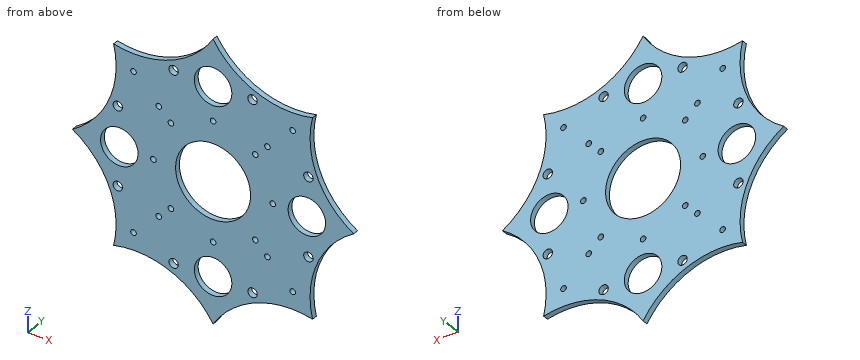
from build123d import *

# Parameters (mm, degrees)
SKETCH_1_R      = 1.5
SKETCH_1_R_2    = 20
SKETCH_1_R_3    = 2.5
SKETCH_1_R_4    = 10
EXTRUDE_2_DEPTH = 3


with BuildPart() as part:
    # 草圖1 → 填料-伸長2 (new body)
    with BuildSketch(Plane(origin=(0, 0, 0), x_dir=(1, 0, 0), z_dir=(0, 1, 0))):
        with BuildLine():
            ThreePointArc((-53.033008589, 53.033008589), (-22.961005942, 55.432771951), (0, 75))
            ThreePointArc((0, 75), (22.961005942, 55.432771951), (53.033008589, 53.033008589))
            ThreePointArc((53.033008589, 53.033008589), (55.432771951, 22.961005942), (75, 0))
            ThreePointArc((75, 0), (55.432771951, -22.961005942), (53.033008589, -53.033008589))
            ThreePointArc((53.033008589, -53.033008589), (22.961005942, -55.432771951), (0, -75))
            ThreePointArc((0, -75), (-22.961005942, -55.432771951), (-53.033008589, -53.033008589))
            ThreePointArc((-53.033008589, -53.033008589), (-55.432771951, -22.961005942), (-75, 0))
            ThreePointArc((-75, 0), (-55.432771951, 22.961005942), (-53.033008589, 53.033008589))
        make_face()
        with Locations(Location((-42.426406871, 42.426406871, 0), (0, 0, 270))):
            Circle(SKETCH_1_R, mode=Mode.SUBTRACT)
        with Locations(Location((-28.991378029, 28.991378029, 0), (0, 0, 270))):
            Circle(SKETCH_1_R, mode=Mode.SUBTRACT)
        with Locations(Location((28.991378029, -28.991378029, 0), (0, 0, 270))):
            Circle(SKETCH_1_R, mode=Mode.SUBTRACT)
        with Locations(Location((42.426406871, -42.426406871, 0), (0, 0, 270))):
            Circle(SKETCH_1_R, mode=Mode.SUBTRACT)
        with Locations(Location((42.426406871, 42.426406871, 0), (0, 0, 270))):
            Circle(SKETCH_1_R, mode=Mode.SUBTRACT)
        with Locations(Location((28.991378029, 28.991378029, 0), (0, 0, 270))):
            Circle(SKETCH_1_R, mode=Mode.SUBTRACT)
        with Locations(Location((-28.991378029, -28.991378029, 0), (0, 0, 270))):
            Circle(SKETCH_1_R, mode=Mode.SUBTRACT)
        with Locations(Location((-42.426406871, -42.426406871, 0), (0, 0, 270))):
            Circle(SKETCH_1_R, mode=Mode.SUBTRACT)
        with Locations(Location((0, 0, 0), (0, 0, 270))):
            Circle(SKETCH_1_R_2, mode=Mode.SUBTRACT)
        with Locations(Location((0, 31.819805153, 0), (0, 0, 270))):
            Circle(SKETCH_1_R, mode=Mode.SUBTRACT)
        with Locations(Location((31.819805153, 0, 0), (0, 0, 270))):
            Circle(SKETCH_1_R, mode=Mode.SUBTRACT)
        with Locations(Location((22.5, 22.5, 0), (0, 0, 270))):
            Circle(SKETCH_1_R, mode=Mode.SUBTRACT)
        with Locations(Location((0, -31.819805153, 0), (0, 0, 270))):
            Circle(SKETCH_1_R, mode=Mode.SUBTRACT)
        with Locations(Location((-22.5, -22.5, 0), (0, 0, 270))):
            Circle(SKETCH_1_R, mode=Mode.SUBTRACT)
        with Locations(Location((-31.819805153, 0, 0), (0, 0, 270))):
            Circle(SKETCH_1_R, mode=Mode.SUBTRACT)
        with Locations(Location((-22.5, 22.5, 0), (0, 0, 270))):
            Circle(SKETCH_1_R, mode=Mode.SUBTRACT)
        with Locations(Location((22.5, -22.5, 0), (0, 0, 270))):
            Circle(SKETCH_1_R, mode=Mode.SUBTRACT)
        with Locations(Location((-21.04758878, 50.813374288, 0), (0, 0, 270))):
            Circle(SKETCH_1_R_3, mode=Mode.SUBTRACT)
        with Locations(Location((21.04758878, 50.813374288, 0), (0, 0, 270))):
            Circle(SKETCH_1_R_3, mode=Mode.SUBTRACT)
        with Locations(Location((50.813374288, 21.04758878, 0), (0, 0, 270))):
            Circle(SKETCH_1_R_3, mode=Mode.SUBTRACT)
        with Locations(Location((50.813374288, -21.04758878, 0), (0, 0, 270))):
            Circle(SKETCH_1_R_3, mode=Mode.SUBTRACT)
        with Locations(Location((21.04758878, -50.813374288, 0), (0, 0, 270))):
            Circle(SKETCH_1_R_3, mode=Mode.SUBTRACT)
        with Locations(Location((-21.04758878, -50.813374288, 0), (0, 0, 270))):
            Circle(SKETCH_1_R_3, mode=Mode.SUBTRACT)
        with Locations(Location((-50.813374288, -21.04758878, 0), (0, 0, 270))):
            Circle(SKETCH_1_R_3, mode=Mode.SUBTRACT)
        with Locations(Location((-50.813374288, 21.04758878, 0), (0, 0, 270))):
            Circle(SKETCH_1_R_3, mode=Mode.SUBTRACT)
        with Locations(Location((0, 50, 0), (0, 0, 270))):
            Circle(SKETCH_1_R_4, mode=Mode.SUBTRACT)
        with Locations(Location((50, 0, 0), (0, 0, 270))):
            Circle(SKETCH_1_R_4, mode=Mode.SUBTRACT)
        with Locations(Location((0, -50, 0), (0, 0, 270))):
            Circle(SKETCH_1_R_4, mode=Mode.SUBTRACT)
        with Locations(Location((-50, 0, 0), (0, 0, 270))):
            Circle(SKETCH_1_R_4, mode=Mode.SUBTRACT)
    extrude(amount=EXTRUDE_2_DEPTH)


solid = part.part
Check sheet for the modelled part. Datum: model origin and axes. Units: mm. Coordinates: 2 decimals unless noted, no trailing zeros. Loops run counter-clockwise (first coordinate to the right, second up) from the corner with the lowest first, then second, coordinate; pieces in that order, holes last. Notation, with made-up numbers: (-13.5, -37) -> (26.5, -37) arc R29 ccw to (26.5, -3) -> close; hole circle Ø5 at (-20.5, 61). An arc over 180 degrees is marked (long way). Answer in a Markdown table with one row per item.
1. Sectioned sample at C-C, the plane y = 1. Give the number of separate pieces and of enclosed holes in the cut face, then the cut area to 3 significant figures.
Check values:
| item | result |
|---|---|
| separate pieces | 1 |
| enclosed holes | 29 |
| area | 10,200 mm2 |
2. Sectioned sample at D-D, the plane x = -35.5. Record the boundary of the cut face in (y, z).
Check values:
| item | result |
|---|---|
| outline | (0, -52.1) -> (3, -52.1) -> (3, 52.1) -> (0, 52.1) -> close |
3. Material ranges on line 1 along Z through (x, y) = (-2, 1.2); line 2 along Z through (x, y) = (9, 0.4); line 3 along Z through (x, y) = (-28, 1.65), recorded low to high. Write a range as [from, to].
Check values:
| item | result |
|---|---|
| line 1 | z = [-72, -59.8], [-40.2, -19.9], [19.9, 40.2], [59.8, 72] |
| line 2 | z = [-64.22, -54.36], [-45.64, -17.86], [17.86, 45.64], [54.36, 64.22] |
| line 3 | z = [-53.66, -30.12], [-27.87, 27.87], [30.12, 53.66] |
4. Sectioned sample at B-B, the plane z = 14.5. Record the boundary of the cut face in (x, y).
Check values:
| item | result |
|---|---|
| outline | (-59.95, 0) -> (-13.77, 0) -> (-13.77, 3) -> (-59.95, 3) -> close; (13.77, 0) -> (59.95, 0) -> (59.95, 3) -> (13.77, 3) -> close |
5. Go/stop test with flat-tipped pins: pin 1 (6.5 mm diameter, centred on x = -50.81, z = 21.05, fed in from +Y); pin 2 (1.8 mm diameter, centred on x = -22.5, z = -22.5, fed in from +Y); pin 3 (1.5 mm diameter, centred on y = 1.5, z = -14, fed in from +X). Record where each tip stops, or that it passes through.
Check values:
| item | result |
|---|---|
| pin 1 | stops at y = 3 |
| pin 2 | passes through |
| pin 3 | stops at x = 60.82 |
6. Sectioned sample at A-A, the plane x = -15. Record the boundary of the cut face in (y, z).
Check values:
| item | result |
|---|---|
| outline | (0, -59.62) -> (3, -59.62) -> (3, -13.23) -> (0, -13.23) -> close; (0, 13.23) -> (3, 13.23) -> (3, 59.62) -> (0, 59.62) -> close |
